from build123d import *

# Parameters (mm, degrees)
SKETCH_1_R          = 7
EXTRUDE_1_DEPTH     = 5
SKETCH_2_R          = 4
EXTRUDE_2_DEPTH     = 2
SKETCH_3_R          = 3
EXTRUDE_3_DEPTH     = 10
CHAMFER_1_SIZE      = 0.2
CUT_EXTRUDE_1_DEPTH = 2.5


with BuildPart() as part:
    # 草图1 → 凸台-拉伸1 (new body)
    with BuildSketch(Plane(origin=(0, 0, 0), x_dir=(1, 0, 0), z_dir=(0, 1, 0))):
        with Locations(Location((0, 0, 0), (0, 0, 270))):
            Circle(SKETCH_1_R)
    extrude(amount=EXTRUDE_1_DEPTH)

    # 草图2 → 凸台-拉伸2 (add)
    with BuildSketch(Plane(origin=(0, 5, 0), x_dir=(1, 0, 0), z_dir=(0, 1, 0))):
        with Locations(Location((0, 0, 0), (0, 0, 270))):
            Circle(SKETCH_2_R)
    extrude(amount=EXTRUDE_2_DEPTH)

    # 草图3 → 凸台-拉伸3 (add)
    with BuildSketch(Plane(origin=(0, 7, 0), x_dir=(1, 0, 0), z_dir=(0, 1, 0))):
        with Locations(Location((0, 0, 0), (0, 0, 270))):
            Circle(SKETCH_3_R)
    extrude(amount=EXTRUDE_3_DEPTH)

    # 倒角1
    chamfer_1_edges = [part.edges().sort_by_distance(p)[0] for p in [
        (0, 17, -3),
        (0, 0, -7),
        (0, 5, -7),
        (0, 7, -4),
    ]]
    chamfer(chamfer_1_edges, length=CHAMFER_1_SIZE)

    # 草图4 → 切除-拉伸1 (cut)
    with BuildSketch(Plane.XZ):
        Polygon((2.886751346, 0), (1.443375673, 2.5), (-1.443375673, 2.5), (-2.886751346, 0), (-1.443375673, -2.5), (1.443375673, -2.5), align=None)
    extrude(amount=-CUT_EXTRUDE_1_DEPTH, mode=Mode.SUBTRACT)


solid = part.part
Geometry check sheet. Reference: the model listing, model coordinates, mm. A direction names the side the tool comes from. Round coordinates to 2 decimals unless told otherwise and drop trailing zeros. Loops run counter-clockwise (first coordinate to the right, second up) from the corner with the lowest first, then second, coordinate; pieces in that order, holes last. Notation, with made-up numbers: (22.25, -20.75) - (54.25, -20.75) arc R21 cw to (54.25, -10.75) - close; hole circle Ø11 at (36, -37). An arc over 180 degrees is marked (long way). One line per question, with ' | ' between items. Start each with the question number.
1. Draft check along Z on faces 1 (the face through (2.175, 1.232, 1.233)), 2 (the face through (0, 0, 3)), 3 (the face through (-3.905, 5.887, -0.867)). Enter one of: released by +Z, released by -Z, zero draft, split by the parting line, or undercut.
2. Scan lines: line 1 (Y direction, x = 5, z = 1.75); line 2 (Y direction, x = 0, z = 3.75); line 3 (X direction, y = 8, z = -2.5). Record each from-to range of solid material in increasing order. Write a range as [from, to].
3. Cross-section at B-B on y = 11.75. Record the cut outline in (x, z).
4. Tool access check on faces 4 (the face through (0, 1, -2.5)), 5 (the face through (-6.834, 2.468, -1.517)), 6 (the face through (0.9, 11.83, 2.86)). Record the directions out of +Z, -Z, +X, -X, +Y, -Y that give a thin tool (end or side, any length) a straight path to the whole face; none if there is none.
5. Cross-section at A-A on x = 0. Record the cut outline in (y, z), then the cut area to 3 significant figures.
6. Depth check by flat-ended pin: pin 1 (6 mm diameter, centred on x = 3.5, z = -5, fed in from +Y); pin 2 (6 mm diameter, centred on x = -4.5, y = 12.5, fed in from +Z); pin 3 (2 mm diameter, centred on x = 3, y = 13.5, fed in from -Z). Enter the tip coordinate at first touch or a pass-through.
Taken from the geometry:
1) face 1: undercut | face 2: zero draft | face 3: split by the parting line
2) line 1: [0, 5] | line 2: [0, 7] | line 3: [-1.66, 1.66]
3) outline: circle Ø6 at (0, 0)
4) face 4: -Y | face 5: +Y, -Y | face 6: +Y
5) outline: (0, -6.8) - (0.2, -7) - (4.8, -7) - (5, -6.8) - (5, -4) - (6.8, -4) - (7, -3.8) - (7, -3) - (16.8, -3) - (17, -2.8) - (17, 2.8) - (16.8, 3) - (7, 3) - (7, 3.8) - (6.8, 4) - (5, 4) - (5, 6.8) - (4.8, 7) - (0.2, 7) - (0, 6.8) - (0, 2.5) - (2.5, 2.5) - (2.5, -2.5) - (0, -2.5) - close | area: 133 mm²
6) pin 1: y = 7 | pin 2: z = 2.6 | pin 3: z = -2.24
